```python
from build123d import *

# Parameters (mm, degrees)
SKETCH_1_W          = 300
SKETCH_1_H          = 360
EXTRUDE_1_DEPTH     = 9
SKETCH_2_W          = 130
SKETCH_2_H          = 260
CUT_EXTRUDE_1_DEPTH = 9
SKETCH_3_R          = 1.5
CUT_EXTRUDE_2_DEPTH = 10
FILLET_1_R          = 20
SKETCH_5_R          = 1.65
SKETCH_5_R_2        = 1.7
CUT_EXTRUDE_4_DEPTH = 10


with BuildPart() as part:
    # 草图1 → 凸台-拉伸1 (new body)
    with BuildSketch(Plane(origin=(0, 0, 0), x_dir=(1, 0, 0), z_dir=(0, 1, 0))):
        Rectangle(SKETCH_1_W, SKETCH_1_H)
    extrude(amount=EXTRUDE_1_DEPTH)

    # 草图2 → 切除-拉伸1 (cut)
    with BuildSketch(Plane(origin=(0, 9, 0), x_dir=(1, 0, 0), z_dir=(0, 1, 0))):
        with Locations((0, 50)):
            Rectangle(SKETCH_2_W, SKETCH_2_H)
    extrude(amount=-CUT_EXTRUDE_1_DEPTH, mode=Mode.SUBTRACT)

    # 草图3 → 切除-拉伸2 (cut)
    with BuildSketch(Plane(origin=(0, 9, 0), x_dir=(1, 0, 0), z_dir=(0, 1, 0))):
        with Locations(Location((-95, 160, 0), (0, 0, 270))):
            Circle(SKETCH_3_R)
        with Locations(Location((-95, 140, 0), (0, 0, 270))):
            Circle(SKETCH_3_R)
        with Locations(Location((95, 140, 0), (0, 0, 270))):
            Circle(SKETCH_3_R)
        with Locations(Location((95, 160, 0), (0, 0, 270))):
            Circle(SKETCH_3_R)
        with Locations(Location((-10, -100, 0), (0, 0, 270))):
            Circle(SKETCH_3_R)
        with Locations(Location((10, -100, 0), (0, 0, 270))):
            Circle(SKETCH_3_R)
    extrude(amount=-CUT_EXTRUDE_2_DEPTH, mode=Mode.SUBTRACT)

    # 圆角1
    fillet_1_edges = [part.edges().sort_by_distance(p)[0] for p in [
        (65, 4.5, -180),
        (-65, 4.5, -180),
        (150, 4.5, 180),
        (-150, 4.5, 180),
        (-150, 4.5, -180),
        (150, 4.5, -180),
    ]]
    fillet(fillet_1_edges, radius=FILLET_1_R)

    # 草图5 → 切除-拉伸4 (cut)
    with BuildSketch(Plane(origin=(0, 9, 0), x_dir=(1, 0, 0), z_dir=(0, 1, 0))):
        with Locations(Location((-113.35, 24.35, 0), (0, 0, 270))):
            Circle(SKETCH_5_R)
        with Locations(Location((-144.35, 24.35, 0), (0, 0, 270))):
            Circle(SKETCH_5_R)
        with Locations(Location((-143.85, 38.85, 0), (0, 0, 270))):
            Circle(SKETCH_5_R_2)
        with Locations(Location((-113.85, 38.85, 0), (0, 0, 270))):
            Circle(SKETCH_5_R_2)
        with Locations(Location((-144.35, -6.65, 0), (0, 0, 270))):
            Circle(SKETCH_5_R)
        with Locations(Location((-143.85, -21.15, 0), (0, 0, 270))):
            Circle(SKETCH_5_R_2)
        with Locations(Location((-113.85, -21.15, 0), (0, 0, 270))):
            Circle(SKETCH_5_R_2)
        with Locations(Location((-113.35, -6.65, 0), (0, 0, 270))):
            Circle(SKETCH_5_R)
    cut_extrude_4 = extrude(amount=-CUT_EXTRUDE_4_DEPTH, mode=Mode.SUBTRACT)

    # 镜向2: 切除-拉伸4 across plane
    add(cut_extrude_4.mirror(Plane(origin=(0, 0, 0), x_dir=(0, 0, 1), z_dir=(1, 0, 0))), mode=Mode.SUBTRACT)


solid = part.part
```
Could you check a few things on this model? Use its own coordinates, in mm. A direction names the side the tool comes from. Round coordinates to 2 decimals unless told otherwise and drop trailing zeros. Loops run counter-clockwise (first coordinate to the right, second up) from the corner with the lowest first, then second, coordinate; pieces in that order, holes last. Notation, with made-up numbers: M 44.25,1.25 L 54.25,1.25 A4 ccw 54.25,7.25 Z; hole C 5,4 d3. An arc over 180 degrees is marked long. Put each result on its own line as item: value.
Q1. Imagine slicing it at A-A (z = -15.5). Write out the boundary of the cut face in (x, y), then the cut area to 3 significant figures.
Check result:
outline: M -150,0 L -65,0 L -65,9 L -150,9 Z; M 65,0 L 150,0 L 150,9 L 65,9 Z
area: 1,530 mm2
Q2. For pin 1 (1 mm diameter, centred on x = 70, y = 5, fed in from -Z) (3 decimals), with a flat end and sliding along its axis, tell me the tip position at first contact or that it passes through.
Check result:
pin 1: z = -173.775
Q3. Imagine slicing it at C-C (x = -18). Write out the boundary of the cut face in (y, z).
Check result:
outline: M 0,80 L 9,80 L 9,180 L 0,180 Z
Q4. On a 3-axis mill with a long thin cutter (end or side, diameter ignored), from which of +Z, -Z, +X, -X, +Y, -Y can I reach the whole of each face in a straight line? I mean faces 1 (the face through (65, 5, -38)), 2 (the face through (-150, 4, 2)). Say none if no direction works.
Check result:
face 1: -Z, +Y, -Y
face 2: +Z, -Z, -X, +Y, -Y
Q5. Thinking about a two-plate mould opening in X: for faces 3 (the face through (-144.297, 4.563, 173.986)), 4 (the face through (-108, 4, -180)), 5 (the face through (71.014, 4.437, -174.297)), which applies, released by +X, released by -X, zero draft, split by the parting line, or undercut?
Check result:
face 3: released by -X
face 4: zero draft
face 5: undercut
Q6. Imagine slicing it at B-B (y = 6.75). State how many separate pieces and enclosed holes the cut face has, then the cut area to 3 significant figures.
Check result:
separate pieces: 1
enclosed holes: 22
area: 73,500 mm2
Q7. I need wall thicknesses on probe 1 along X at (y, z) = (3, 6.65); probe 2 along X at (y, z) = (3, -38.85); probe 3 along X at (y, z) = (6.5, -160). Which ranges of each line are inside material? Lowest first, please.
Check result:
probe 1: -150 to -146, -142.7 to -115, -111.7 to -65, 65 to 111.7, 115 to 142.7, 146 to 150
probe 2: -150 to -145.55, -142.15 to -115.55, -112.15 to -65, 65 to 112.15, 115.55 to 142.15, 145.55 to 150
probe 3: -150 to -96.5, -93.5 to -65, 65 to 93.5, 96.5 to 150
